CAD build for the part. Positions are in the model's coordinates, mm. Face numbers are marked on the shaded views. A direction names the side the tool comes from. Give positions to 0.01 mm unless a question says otherwise; leave off trailing zeros. Loops run counter-clockwise (first coordinate to the right, second up) from the corner with the lowest first, then second, coordinate; pieces in that order, holes last. Notation, with made-up numbers: (83.5, -10.5) - (110.5, -10.5) arc R19 cw to (110.5, 18.5) - close; hole circle Ø4 at (72, -13). An arc over 180 degrees is marked (long way). Return JSON: item names as keys, results as strings.
from build123d import *

# Parameters (mm, degrees)
F1_DEPTH = 105
F2_T     = -5
F4_DEPTH = 95
F6_D     = 5


with BuildPart() as f1:
    # F0 (on Front) → F1 (new body)
    with BuildSketch(Plane.XZ):
        Polygon((74.5727300216, 75.5225419998), (-75.4272699784, 75.5225419998), (-0.4272699784, -54.3812685678), align=None)
    extrude(amount=F1_DEPTH)

    # F2
    f2_openings = [f1.faces().sort_by_distance(p)[0] for p in [
        (-0.42727, -52.5, 75.522542),
    ]]
    offset(amount=F2_T, openings=f2_openings)

    # F3 (on face) → F4 (join)
    with BuildSketch(Plane.XZ.offset(5)):
        Polygon((44.5727300216, 33.5610177728), (-60.4272699784, 59.5417798863), (-0.4272699784, -44.3812685678), align=None)
    extrude(amount=F4_DEPTH)

    # F6 (through all)
    with Locations(Plane(origin=(18.8972005322, 0, -10.9103038142), x_dir=(0, -1, 0), z_dir=(-0.8660254038, 0, 0.5))):
        with Locations((92.5, 56.3510589789), (82.5, 56.3510589789), (72.5, 56.3510589789), (62.5, 56.3510589789), (52.5, 56.3510589789), (42.5, 56.3510589789), (32.5, 56.3510589789), (22.5, 56.3510589789), (12.5, 56.3510589789)):
            Hole(F6_D / 2)


solid = f1.part
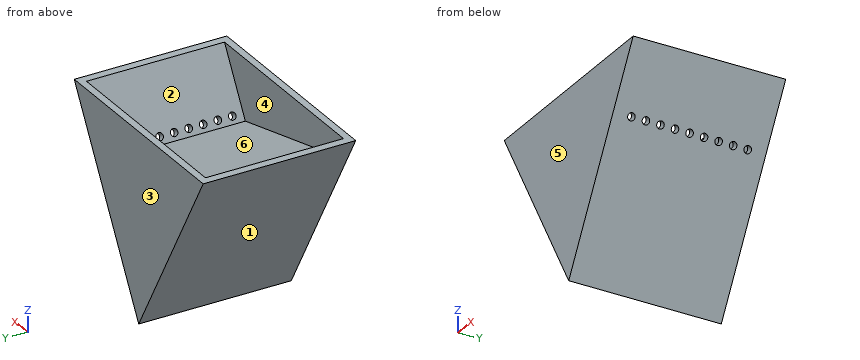
1. Cut at D-D, the plane z = -26. Write the cut outline in (x, y).
Values follow:
{"outline": "(-16.81, -105) - (15.96, -105) - (15.96, 0) - (-16.81, 0) - close"}
2. Cut at C-C, the plane z = 67.5. Write the cut outline in (x, y), plus the area to 3 significant figures.
Values follow:
{"outline": "(-70.8, -105) - (69.94, -105) - (69.94, 0) - (-70.8, 0) - close; hole (-65.02, -100) - (64.17, -100) - (64.17, -5) - (-65.02, -5) - close", "area": "2,500 mm²"}
3. Which spindle directions (+Z, -Z, +X, -X, +Y, -Y) get a long thin tool onto all of the face, cutting with end or side? Do the marked faces 1 and 2. Say none if no direction does.
Values follow:
{"face 1": "-Z, -X, +Y, -Y", "face 2": "+Z"}
4. Drill centre lines: probe 1 along Y at (x, z) = (-33, 53.5); probe 2 along X at (y, z) = (-18, 67.5); probe 3 along X at (y, z) = (-80, 28). Where is each one in solid material? Low to high.
Values follow:
{"probe 1": "y = -105 to -100, -5 to 0", "probe 2": "x = -70.8 to -65.02, 64.17 to 69.94", "probe 3": "x = -47.99 to 47.14"}
5. Cut at B-B, the plane x = -62.5. Write the cut outline in (y, z).
Values follow:
{"outline": "(-105, 53.13) - (0, 53.13) - (0, 75.52) - (-5, 75.52) - (-5, 63.13) - (-100, 63.13) - (-100, 75.52) - (-105, 75.52) - close"}
6. Cut at A-A, the plane y = -62.5. Write the cut outline in (x, z), plus the area to 3 significant figures.
Values follow:
{"outline": "(-75.43, 75.52) - (-0.43, -54.38) - (50.15, 33.23) - (45.82, 35.73) - (44.57, 33.56) - (-60.43, 59.54) - (-69.65, 75.52) - close; (48.32, 40.06) - (52.65, 37.56) - (74.57, 75.52) - (68.8, 75.52) - close", "area": "6,090 mm²"}
7. Drop flat-ended pins along their axis: P1, Ø8, axis at x = 4, y = -18.5, coming from the -Z side; P2, Ø2, axis at y = -11, z = 4.5, coming from the -X side; P3, Ø2, axis at x = 22.5, y = -91.5, coming from the +Z side. Give the stop position or say it passes through.
Values follow:
{"P1": "stops at z = -53.64", "P2": "stops at x = -35", "P3": "stops at z = 39.27"}
8. Pull direction Y, two halves, no side cores. Call the marked faces 3, 4, 5 and 6: +Y half, -Y half, draft (parallel to the pull), parting line (faces both ways), or undercut.
Values follow:
{"face 3": "+Y half", "face 4": "undercut", "face 5": "-Y half", "face 6": "undercut"}
